Verification items for the finished model (mm, model axes). Face numbers are marked on the shaded views. A direction names the side the tool comes from. Coordinates: 2 decimals unless noted, no trailing zeros. Loops run counter-clockwise (first coordinate to the right, second up) from the corner with the lowest first, then second, coordinate; pieces in that order, holes last. Notation, with made-up numbers: (79, -31) - (93, -31) arc R21 cw to (93, 6) - close; hole circle Ø10 at (-18.75, 23.5). An arc over 180 degrees is marked (long way). Answer as CSV lines item,"result". Start each with the question number.
1. Cross-section at B-B (y = 9.8). Enter the section's corners in (x, z).
2. Cross-section at A-A (z = 27.5). Enter the section's corners in (x, y), plus the area to 3 significant figures.
3. Set-up check for the marked faces 1, 2 and 3: record each of +Z, -Z, +X, -X, +Y, -Y from which the full face is reachable in a straight line by a thin tool's end or side.
4. Material ranges on line 1 (X direction, y = 17.75, z = 12); line 2 (Z direction, x = 38, y = 2.5); line 3 (Z direction, x = 10, y = 14), recorded low to high. Write a range as [from, to].
5. Cross-section at C-C (x = -4). Enter the section's corners in (y, z).
6. Gauge pin test, flat ends, axial feed: P1, Ø1, axis at x = -6, z = 28, coming from the +Y side; P2, Ø0.6, axis at x = 46.5, z = 27.5, coming from the -Y side; P3, Ø10, axis at x = 19.5, y = 12, coming from the +Z side. Record the tip position at first contact, or that the pin passes through.
7. Cross-section at D-D (x = 5). Enter the section's corners in (y, z).
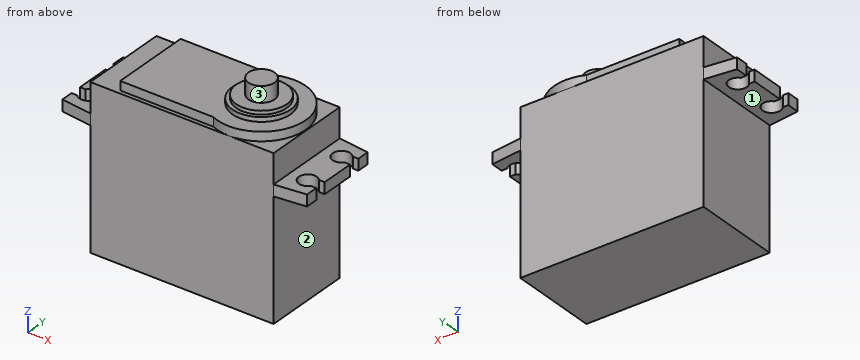
```python
from build123d import *

# Parameters (mm, degrees)
SKETCH_1_W          = 40.6
SKETCH_1_H          = 19.6
EXTRUDE_1_DEPTH     = 35.5
SKETCH_2_R          = 9.8
EXTRUDE_2_DEPTH     = 2
SKETCH_3_W          = 20.607820144
SKETCH_3_H          = 17.9
EXTRUDE_3_DEPTH     = 2
SKETCH_4_R          = 6.45
EXTRUDE_4_DEPTH     = 1
SKETCH_5_R          = 5.6
EXTRUDE_5_DEPTH     = 0.8
SKETCH_7_R          = 2.9
EXTRUDE_6_DEPTH     = 3.5
EXTRUDE_7_DEPTH     = 2.5
CUT_EXTRUDE_1_REACH = 31
SKETCH_9_R          = 2
CUT_EXTRUDE_2_REACH = 31
SKETCH_10_W         = 1.6
SKETCH_10_H         = 2.5


with BuildPart() as part:
    # ｽｹｯﾁ1 → ﾎﾞｽ - 押し出し1 (new body)
    with BuildSketch(Plane.XY):
        with Locations((20.3, 9.8)):
            Rectangle(SKETCH_1_W, SKETCH_1_H)
    extrude(amount=EXTRUDE_1_DEPTH)

    # ｽｹｯﾁ2 → ﾎﾞｽ - 押し出し2 (add)
    with BuildSketch(Plane.XY.offset(35.5)):
        with Locations((30.6, 9.8)):
            Circle(SKETCH_2_R)
    extrude(amount=EXTRUDE_2_DEPTH)

    # ｽｹｯﾁ3 → ﾎﾞｽ - 押し出し3 (add)
    with BuildSketch(Plane.XY.offset(35.5)):
        with Locations((16.303910072, 9.8)):
            Rectangle(SKETCH_3_W, SKETCH_3_H)
    extrude(amount=EXTRUDE_3_DEPTH)

    # ｽｹｯﾁ4 → ﾎﾞｽ - 押し出し4 (add)
    with BuildSketch(Plane.XY.offset(37.5)):
        with Locations((30.6, 9.8)):
            Circle(SKETCH_4_R)
    extrude(amount=EXTRUDE_4_DEPTH)

    # ｽｹｯﾁ5 → ﾎﾞｽ - 押し出し5 (add)
    with BuildSketch(Plane.XY.offset(38.5)):
        with Locations((30.6, 9.8)):
            Circle(SKETCH_5_R)
    extrude(amount=EXTRUDE_5_DEPTH)

    # ｽｹｯﾁ7 → ﾎﾞｽ - 押し出し6 (add)
    with BuildSketch(Plane.XY.offset(39.3)):
        with Locations((30.6, 9.8)):
            Circle(SKETCH_7_R)
    extrude(amount=EXTRUDE_6_DEPTH)

    # ｽｹｯﾁ8 → ﾎﾞｽ - 押し出し7 (add)
    with BuildSketch(Plane.XY.offset(26.5)):
        Polygon((0, 0), (-6.8, 0.8), (-6.8, 18.8), (0, 19.6), align=None)
        Polygon((40.6, 19.6), (40.6, 0), (47.4, 0.8), (47.4, 18.8), align=None)
    extrude(amount=EXTRUDE_7_DEPTH)

    # ｽｹｯﾁ9 → ｶｯﾄ - 押し出し1 (cut, up to next)
    with BuildSketch(Plane.XY.offset(29), mode=Mode.PRIVATE) as cut_extrude_1_sk1:
        with Locations((-4, 4.8)):
            Circle(SKETCH_9_R)
    cut_extrude_1_tool1 = extrude(cut_extrude_1_sk1.sketch, amount=-CUT_EXTRUDE_1_REACH, mode=Mode.PRIVATE) & part.part
    add(cut_extrude_1_tool1.solids().sort_by_distance((-4, 4.8, 29))[0], mode=Mode.SUBTRACT)
    # ｽｹｯﾁ9 → ｶｯﾄ - 押し出し1 (cut, up to next)
    with BuildSketch(Plane.XY.offset(29), mode=Mode.PRIVATE) as cut_extrude_1_sk2:
        with Locations((-4, 14.8)):
            Circle(SKETCH_9_R)
    cut_extrude_1_tool2 = extrude(cut_extrude_1_sk2.sketch, amount=-CUT_EXTRUDE_1_REACH, mode=Mode.PRIVATE) & part.part
    add(cut_extrude_1_tool2.solids().sort_by_distance((-4, 14.8, 29))[0], mode=Mode.SUBTRACT)
    # ｽｹｯﾁ9 → ｶｯﾄ - 押し出し1 (cut, up to next)
    with BuildSketch(Plane.XY.offset(29), mode=Mode.PRIVATE) as cut_extrude_1_sk3:
        with Locations((44.6, 14.8)):
            Circle(SKETCH_9_R)
    cut_extrude_1_tool3 = extrude(cut_extrude_1_sk3.sketch, amount=-CUT_EXTRUDE_1_REACH, mode=Mode.PRIVATE) & part.part
    add(cut_extrude_1_tool3.solids().sort_by_distance((44.6, 14.8, 29))[0], mode=Mode.SUBTRACT)
    # ｽｹｯﾁ9 → ｶｯﾄ - 押し出し1 (cut, up to next)
    with BuildSketch(Plane.XY.offset(29), mode=Mode.PRIVATE) as cut_extrude_1_sk4:
        with Locations((44.6, 4.8)):
            Circle(SKETCH_9_R)
    cut_extrude_1_tool4 = extrude(cut_extrude_1_sk4.sketch, amount=-CUT_EXTRUDE_1_REACH, mode=Mode.PRIVATE) & part.part
    add(cut_extrude_1_tool4.solids().sort_by_distance((44.6, 4.8, 29))[0], mode=Mode.SUBTRACT)

    # ｽｹｯﾁ10 → ｶｯﾄ - 押し出し2 (cut, up to next)
    with BuildSketch(Plane.XY.offset(29), mode=Mode.PRIVATE) as cut_extrude_2_sk1:
        with Locations((-6, 4.8)):
            Rectangle(SKETCH_10_W, SKETCH_10_H)
    cut_extrude_2_tool1 = extrude(cut_extrude_2_sk1.sketch, amount=-CUT_EXTRUDE_2_REACH, mode=Mode.PRIVATE) & part.part
    add(cut_extrude_2_tool1.solids().sort_by_distance((-6, 4.8, 29))[0], mode=Mode.SUBTRACT)
    # ｽｹｯﾁ10 → ｶｯﾄ - 押し出し2 (cut, up to next)
    with BuildSketch(Plane.XY.offset(29), mode=Mode.PRIVATE) as cut_extrude_2_sk2:
        with Locations((-6, 14.8)):
            Rectangle(SKETCH_10_W, SKETCH_10_H)
    cut_extrude_2_tool2 = extrude(cut_extrude_2_sk2.sketch, amount=-CUT_EXTRUDE_2_REACH, mode=Mode.PRIVATE) & part.part
    add(cut_extrude_2_tool2.solids().sort_by_distance((-6, 14.8, 29))[0], mode=Mode.SUBTRACT)
    # ｽｹｯﾁ10 → ｶｯﾄ - 押し出し2 (cut, up to next)
    with BuildSketch(Plane.XY.offset(29), mode=Mode.PRIVATE) as cut_extrude_2_sk3:
        with Locations((46.6, 14.8)):
            Rectangle(SKETCH_10_W, SKETCH_10_H)
    cut_extrude_2_tool3 = extrude(cut_extrude_2_sk3.sketch, amount=-CUT_EXTRUDE_2_REACH, mode=Mode.PRIVATE) & part.part
    add(cut_extrude_2_tool3.solids().sort_by_distance((46.6, 14.8, 29))[0], mode=Mode.SUBTRACT)
    # ｽｹｯﾁ10 → ｶｯﾄ - 押し出し2 (cut, up to next)
    with BuildSketch(Plane.XY.offset(29), mode=Mode.PRIVATE) as cut_extrude_2_sk4:
        with Locations((46.6, 4.8)):
            Rectangle(SKETCH_10_W, SKETCH_10_H)
    cut_extrude_2_tool4 = extrude(cut_extrude_2_sk4.sketch, amount=-CUT_EXTRUDE_2_REACH, mode=Mode.PRIVATE) & part.part
    add(cut_extrude_2_tool4.solids().sort_by_distance((46.6, 4.8, 29))[0], mode=Mode.SUBTRACT)


solid = part.part
```
Values follow:
1,outline,"(-6.8, 26.5) - (0, 26.5) - (0, 0) - (40.6, 0) - (40.6, 26.5) - (47.4, 26.5) - (47.4, 29) - (40.6, 29) - (40.6, 35.5) - (40.4, 35.5) - (40.4, 37.5) - (37.05, 37.5) - (37.05, 38.5) - (36.2, 38.5) - (36.2, 39.3) - (33.5, 39.3) - (33.5, 42.8) - (27.7, 42.8) - (27.7, 39.3) - (25, 39.3) - (25, 38.5) - (24.15, 38.5) - (24.15, 37.5) - (6, 37.5) - (6, 35.5) - (0, 35.5) - (0, 29) - (-6.8, 29) - close"
2,outline,"(-6.8, 0.8) - (0, 0) - (40.6, 0) - (47.4, 0.8) - (47.4, 3.55) - (46.16, 3.55) arc R2 cw (long way) to (46.16, 6.05) - (47.4, 6.05) - (47.4, 13.55) - (46.16, 13.55) arc R2 cw (long way) to (46.16, 16.05) - (47.4, 16.05) - (47.4, 18.8) - (40.6, 19.6) - (0, 19.6) - (-6.8, 18.8) - (-6.8, 16.05) - (-5.56, 16.05) arc R2 cw (long way) to (-5.56, 13.55) - (-6.8, 13.55) - (-6.8, 6.05) - (-5.56, 6.05) arc R2 cw (long way) to (-5.56, 3.55) - (-6.8, 3.55) - close"
2,area,"992 mm²"
3,face 1,"-Z, -X, +Y, -Y"
3,face 2,"-Z, +X, +Y, -Y"
3,face 3,"+Z"
4,line 1,"x = [0, 40.6]"
4,line 2,"z = [0, 35.5]"
4,line 3,"z = [0, 37.5]"
5,outline,"(0.47, 26.5) - (2.8, 26.5) - (2.8, 29) - (0.47, 29) - close; (6.8, 26.5) - (12.8, 26.5) - (12.8, 29) - (6.8, 29) - close; (16.8, 26.5) - (19.13, 26.5) - (19.13, 29) - (16.8, 29) - close"
6,P1,"stops at y = 18.95"
6,P2,"stops at y = 0.66"
6,P3,"stops at z = 38.5"
7,outline,"(0, 0) - (19.6, 0) - (19.6, 35.5) - (0, 35.5) - close"
